Geometry: see drawing. Coordinates: mm, zero at the bounding-box minimum. A direction names the side the tool comes from. Give positions to 0.01 mm unless a question says otherwise; leave off trailing zeros. Loops run counter-clockwise (first coordinate to the right, second up) from the corner with the lowest first, then second, coordinate; pieces in that order, holes last. Notation, with made-up numbers: (-13.5, -6.5) - (13.5, -6.5) arc R19 cw to (13.5, 0.5) - close; hole circle Ø11 at (42.5, 65.5). An arc over 180 degrees is marked (long way). One line per question, with ' | ' between items. Start each with the question number.
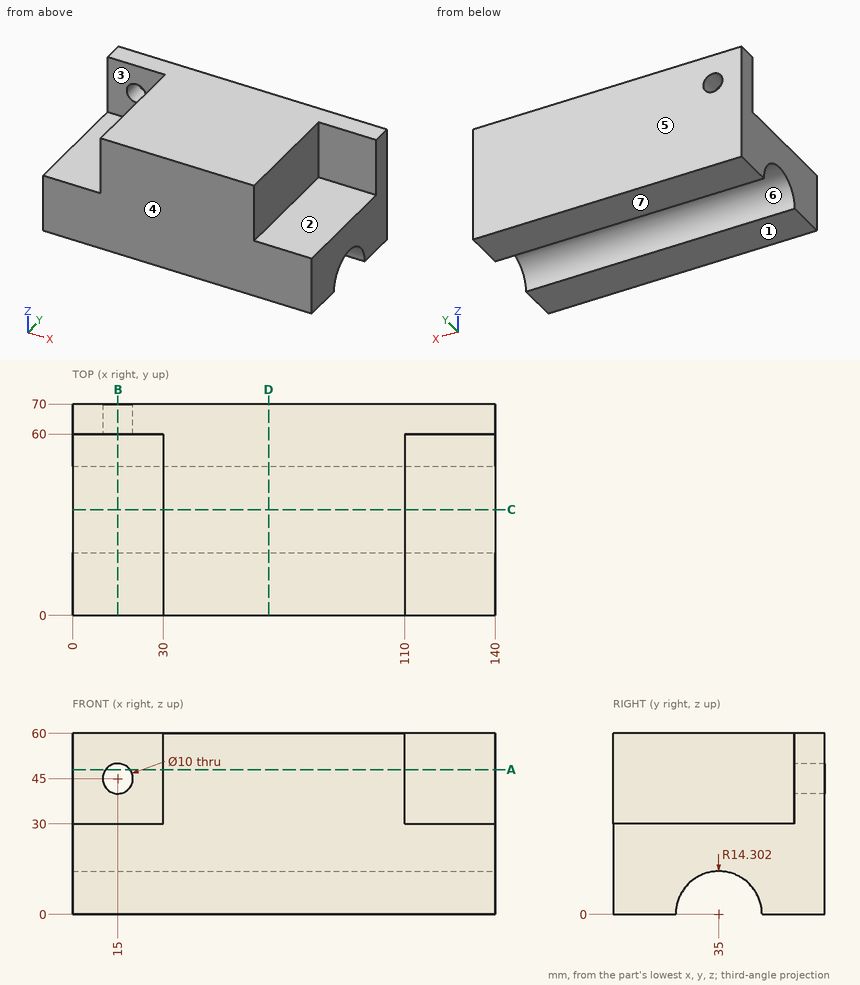
Q1. Access query for the marked faces 1, 2 and 3. Directions: +Z, -Z, +X, -X, +Y, -Y. A direction counts if a zero-diameter tool reaches every point of the face in a straight line with its end or side. Return the directions, or none.
Q2. Section D-D, the plane x = 65. Output: boundary loops of the cut face in (y, z), plus the area to 3 significant figures.
Q3. Section C-C, the plane y = 35. Output: boundary loops of the cut face in (x, z).
Q4. First-contact query: pin 1 (9 mm diameter, centred on x = 7.5, z = 46, fed in from -Y); pin 2 (24 mm diameter, centred on y = 28.5, z = 52.5, fed in from +X). Flat tips, straight axial feed; report the tip coordinate or a pass-through.
Q5. Draft query along Y for the marked faces 4, 5, 6 and 7. Return one class per face: +Y half, -Y half, draft (parallel to the pull), parting line (faces both ways), or undercut.
Q6. Line query: L1, parallel to Z at x = 15, y = 62; L2, parallel to Z at x = 27, y = 16; L3, parallel to X at y = 7, z = 40. Output: solid intervals per line, ascending. Write a range as from..to.
Q7. Section A-A, the plane z = 48. Output: boundary loops of the cut face in (x, y).
Q8. Section B-B, the plane x = 15. Output: boundary loops of the cut face in (y, z), plus the area to 3 significant figures.
Solved:
1) face 1: -Z, +X, -X, +Y, -Y | face 2: +Z, +X, -Y | face 3: +Z, -X, -Y
2) outline: (0, 0) - (20.7, 0) arc R14.3 cw to (49.3, 0) - (70, 0) - (70, 60) - (0, 60) - close | area: 3,880 mm²
3) outline: (0, 14.3) - (140, 14.3) - (140, 30) - (110, 30) - (110, 60) - (30, 60) - (30, 30) - (0, 30) - close
4) pin 1: stops at y = 60 | pin 2: stops at x = 110
5) face 4: -Y half | face 5: +Y half | face 6: undercut | face 7: draft
6) L1: z = 0..40, 50..60 | L2: z = 0..30 | L3: x = 30..110
7) outline: (0, 60) - (11, 60) - (11, 70) - (0, 70) - close; (19, 60) - (30, 60) - (30, 0) - (110, 0) - (110, 60) - (140, 60) - (140, 70) - (19, 70) - close
8) outline: (0, 0) - (20.7, 0) arc R14.3 cw to (49.3, 0) - (70, 0) - (70, 40) - (60, 40) - (60, 30) - (0, 30) - close; (60, 50) - (70, 50) - (70, 60) - (60, 60) - close | area: 1,980 mm²
